from build123d import *

# Parameters (mm, degrees)
SKETCH1_R           = 25
SKETCH1_R_2         = 8
SKETCH1_R_3         = 2
BOSS_EXTRUDE1_DEPTH = 2


with BuildPart() as part:
    # Sketch1 → Boss-Extrude1 (new body)
    with BuildSketch(Plane.XY):
        Circle(SKETCH1_R)
        Circle(SKETCH1_R_2, mode=Mode.SUBTRACT)
        with Locations((-8, 8)):
            Circle(SKETCH1_R_3, mode=Mode.SUBTRACT)
        with Locations((8, 8)):
            Circle(SKETCH1_R_3, mode=Mode.SUBTRACT)
        with Locations(Location((8, -8, 0), (0, 0, 180))):
            Circle(SKETCH1_R_3, mode=Mode.SUBTRACT)
        with Locations(Location((-8, -8, 0), (0, 0, 180))):
            Circle(SKETCH1_R_3, mode=Mode.SUBTRACT)
        with Locations((0, 20.5)):
            Circle(SKETCH1_R_3, mode=Mode.SUBTRACT)
        with Locations((20.5, 0)):
            Circle(SKETCH1_R_3, mode=Mode.SUBTRACT)
        with Locations((0, -20.5)):
            Circle(SKETCH1_R_3, mode=Mode.SUBTRACT)
        with Locations((-20.5, 0)):
            Circle(SKETCH1_R_3, mode=Mode.SUBTRACT)
    extrude(amount=BOSS_EXTRUDE1_DEPTH)


solid = part.part
Check sheet for the modelled part. Datum: model origin and axes. Units: mm. Give positions to 0.01 mm unless a question says otherwise; leave off trailing zeros. Write each loop counter-clockwise with the first axis right and the second up, starting at its lowest first coordinate (ties: lowest second). Pieces come first, ordered by that corner, then holes. Notation, with made-up numbers: (60.5, -14.75) -> (90.5, -14.75) arc R9 cw to (90.5, -6.75) -> close; hole circle Ø10 at (86, 49.25). An arc over 180 degrees is marked (long way). Write item = value, one per line.
Item 1: Release check for a two-part mould opening along X. For faces 1 (the flat face through (-6, 6, 0)), 2 (the cylindrical face through (6.526, 9.352, 0.986)), 3 (the cylindrical face through (23.846, 7.509, 0.986)) record: +X half, -X half, draft (parallel to the pull), parting line (faces both ways), or undercut.
Output:
face_1 = draft
face_2 = undercut
face_3 = parting line
Item 2: Sectioned sample at B-B on z = 1.3. Count the separate pieces of the cut face and the enclosed holes in it, and give its area (3 significant figures).
Output:
separate_pieces = 1
enclosed_holes = 9
area = 1,660 mm^2
Item 3: Sectioned sample at D-D on x = 20.5. Record the boundary of the cut face in (y, z).
Output:
outline = (-14.31, 0) -> (-2, 0) -> (-2, 2) -> (-14.31, 2) -> close; (2, 0) -> (14.31, 0) -> (14.31, 2) -> (2, 2) -> close
Item 4: Sectioned sample at A-A on x = 0. Record the boundary of the cut face in (y, z), and give its area (3 significant figures).
Output:
outline = (-25, 0) -> (-22.5, 0) -> (-22.5, 2) -> (-25, 2) -> close; (-18.5, 0) -> (-8, 0) -> (-8, 2) -> (-18.5, 2) -> close; (8, 0) -> (18.5, 0) -> (18.5, 2) -> (8, 2) -> close; (22.5, 0) -> (25, 0) -> (25, 2) -> (22.5, 2) -> close
area = 52.0 mm^2
Item 5: Scan lines: probe 1 along Y at (x, z) = (0, 0.9); probe 2 along X at (y, z) = (-0.5, 1.8) (1 decimal); probe 3 along X at (y, z) = (-7, 1.7). Record each from-to range of solid material in increasing order. Write a range as from..to.
Output:
probe_1 = -25..-22.5, -18.5..-8, 8..18.5, 22.5..25
probe_2 = -25..-22.4, -18.6..-8, 8..18.6, 22.4..25
probe_3 = -24..-9.73, -6.27..-3.87, 3.87..6.27, 9.73..24
